Part model, mm, in its own coordinate system. A direction names the side the tool comes from. Coordinates: 2 decimals unless noted, no trailing zeros. Loops run counter-clockwise (first coordinate to the right, second up) from the corner with the lowest first, then second, coordinate; pieces in that order, holes last. Notation, with made-up numbers: M 79.5,17 L 137.5,17 A27 ccw 137.5,48 Z; hole C -30,87.25 d11. An arc over 180 degrees is marked long. Answer as CSV lines item,"result". Start each with the question number.
from build123d import *

# Parameters (mm, degrees)
SHELL1_T           = -7.5
SKETCH2_R          = 28.25
SKETCH2_R_2        = 24
CUT_EXTRUDE1_DEPTH = 2
SKETCH4_R          = 3.75
CUT_EXTRUDE2_DEPTH = 75


with BuildPart() as part:
    # Sketch1 → Revolve1 (revolve)
    with BuildSketch(Plane.XY, mode=Mode.PRIVATE) as revolve1_sk:
        Polygon((0, 0), (0, 88), (0, 128), (-63.486315613, 128), (-63.486315613, 108), (-30, 50), (-30, 0), align=None)
    revolve(revolve1_sk.sketch.rotate(Axis((0, 0, 0), (0, 1, 0)), 270), axis=Axis((0, 0, 0), (0, 1, 0)))

    # Shell1
    shell1_openings = [part.faces().sort_by_distance(p)[0] for p in [
        (0, 0, 0),
    ]]
    offset(amount=SHELL1_T, openings=shell1_openings, kind=Kind.INTERSECTION)

    # Sketch2 → Cut-Extrude1 (cut)
    with BuildSketch(Plane.XZ):
        with Locations(Location((0, 0, 0), (0, 0, 270))):
            Circle(SKETCH2_R)
        with Locations(Location((0, 0, 0), (0, 0, 270))):
            Circle(SKETCH2_R_2, mode=Mode.SUBTRACT)
    extrude(amount=-CUT_EXTRUDE1_DEPTH, mode=Mode.SUBTRACT)

    # Sketch4 → Cut-Extrude2 (cut, symmetric)
    with BuildSketch(Plane.XY):
        with Locations((0, 118)):
            Circle(SKETCH4_R)
    extrude(amount=CUT_EXTRUDE2_DEPTH, both=True, mode=Mode.SUBTRACT)


solid = part.part
Q1. Two-plate mould, pull along Y, no slides. Class faces 1 (the face through (-21, 2, 13)), 2 (the face through (-24, 120.5, -1)), 3 (the face through (8.618, 25.641, -20.784)), 4 (the face through (-1, 128, -1)): +Y half, -Y half, draft (parallel to the pull), parting line (faces both ways), or undercut.
Q2. Slice it at A-A, the plane x = 0. Write the cut outline in (y, z).
Q3. Slice it at B-B, the plane z = 0. Write the cut outline in (x, y).
Q4. Slice it at D-D, the plane y = 20. Write the cut outline in (x, z).
Q5. Tool access for faces 5 (the face through (-16.82, 115.18, -53.4)), 6 (the face through (-1.32, 24.65, 29.97)), 7 (the face through (18, 0, -22)): list every direction of +Z, -Z, +X, -X, +Y, -Y with a clear straight run to the whole face (end or side of a thin tool).
Q6. Flat gauge pins, fed straight in: P1, Ø1.5, axis at x = 19.5, z = 15.5, coming from the -Y side; P2, Ø4, axis at x = -34, z = 8, coming from the -Y side; P3, Ø8.5, axis at x = 0, y = 118, coming from the -Z side; P4, Ø2, axis at x = 28, z = -18, coming from the -Y side. Where does each tip first touch, or does it go through?
Q7. Wall check: L1, parallel to X at y = 13, z = 0; L2, parallel to Y at x = 5.5, z = 43.5; L3, parallel to Y at x = 0, z = 13. Give the ranges that are in metal, low to high.
Solved:
1,face 1,"-Y half"
1,face 2,"undercut"
1,face 3,"draft"
1,face 4,"+Y half"
2,outline,"M 0,-30 L 50,-30 L 108,-63.49 L 114.25,-63.49 L 114.25,-55.99 L 110.01,-55.99 L 52.01,-22.5 L 0,-22.5 L 0,-24 L 2,-24 L 2,-28.25 L 0,-28.25 Z; M 0,22.5 L 52.01,22.5 L 110.01,55.99 L 114.25,55.99 L 114.25,63.49 L 108,63.49 L 50,30 L 0,30 L 0,28.25 L 2,28.25 L 2,24 L 0,24 Z; M 121.75,-63.49 L 128,-63.49 L 128,63.49 L 121.75,63.49 Z"
3,outline,"M -63.49,108 L -30,50 L -30,0 L -28.25,0 L -28.25,2 L -24,2 L -24,0 L -22.5,0 L -22.5,52.01 L -55.99,110.01 L -55.99,120.5 L -2.8,120.5 A3.75 cw 2.8,120.5 L 55.99,120.5 L 55.99,110.01 L 22.5,52.01 L 22.5,0 L 24,0 L 24,2 L 28.25,2 L 28.25,0 L 30,0 L 30,50 L 63.49,108 L 63.49,128 L -63.49,128 Z"
4,outline,"C 0,0 d60; hole C 0,0 d45"
5,face 5,"none"
5,face 6,"-Y"
5,face 7,"+Z, -Z, +X, -X, -Y"
6,P1,"stops at y = 2"
6,P2,"stops at y = 55.07"
6,P3,"stops at z = -63.49"
6,P4,"stops at y = 53.96"
7,L1,"x = -30 to -22.5, 22.5 to 30"
7,L2,"y = 73.98 to 88.98, 120.5 to 128"
7,L3,"y = 121.75 to 128"
